from build123d import *

# Parameters (mm, degrees)
SKETCH1_R             = 20
SKETCH1_R_2           = 15
BOSS_EXTRUDE1_DEPTH   = 60
BOSS_EXTRUDE1_2_DEPTH = 60
BOSS_EXTRUDE2_START   = -50
BOSS_EXTRUDE2_DEPTH   = 40


with BuildPart() as part:
    # Sketch1 → Boss-Extrude1 (new body)
    with BuildSketch(Plane.XY):
        Circle(SKETCH1_R)
        Circle(SKETCH1_R_2, mode=Mode.SUBTRACT)
    extrude(amount=BOSS_EXTRUDE1_DEPTH)



with BuildPart() as body_2:
    # Sketch1 → Boss-Extrude1 2 (new body)
    with BuildSketch(Plane.XY):
        with Locations((390, 0)):
            Circle(SKETCH1_R)
        with Locations((390, 0)):
            Circle(SKETCH1_R_2, mode=Mode.SUBTRACT)
    extrude(amount=BOSS_EXTRUDE1_2_DEPTH)


with BuildPart() as part_1:
    add(part.part)

    add(body_2.part)  # Boss-Extrude2 merges body 2
    # Sketch2 → Boss-Extrude2 (add)
    with BuildSketch(Plane.XY.offset(60).offset(BOSS_EXTRUDE2_START)):
        with BuildLine():
            Line((0, -30), (390, -30))
            ThreePointArc((390, -30), (420, 0), (390, 30))
            Line((390, 30), (0, 30))
            ThreePointArc((0, 30), (-30, 0), (0, -30))
        make_face()
        with BuildLine():
            Line((0, 20), (390, 20))
            ThreePointArc((390, 20), (410, 0), (390, -20))
            Line((390, -20), (0, -20))
            ThreePointArc((0, -20), (-20, 0), (0, 20))
        make_face(mode=Mode.SUBTRACT)
    extrude(amount=BOSS_EXTRUDE2_DEPTH)


solid = part_1.part
Build history of the part. All positions in model axes, mm. A direction names the side the tool comes from. Round coordinates to 2 decimals unless told otherwise and drop trailing zeros. Write each loop counter-clockwise with the first axis right and the second up, starting at its lowest first coordinate (ties: lowest second). Pieces come first, ordered by that corner, then holes. Notation, with made-up numbers: M -12,80.5 L 46,80.5 A20 ccw 46,100.5 Z; hole C 7,33.5 d1. An arc over 180 degrees is marked long. Answer as a JSON object with one key per item and string values. Group by question number.
(1) Cut at C-C (y = 0). Give the cut face in (x, z), and give its area (3 significant figures).
(2) Flat gauge pins, fed straight in: pin 1 (6 mm diameter, centred on y = 13.5, z = 25.5, fed in from -X); pin 2 (6 mm diameter, centred on y = 6.5, z = 49, fed in from -X); pin 3 (1.5 mm diameter, centred on x = 270, y = -20.5, fed in from +Z). Where does each tip first touch, or does it go through?
(3) Cut at A-A (x = 97.5). Give the cut face in (y, z).
(4) Mould opens along X. For faces 3 (the cylindrical face through (-14.985, 0.66, 29.58)), 4 (the flat face through (198, 30, 30)), 5 (the cylindrical face through (-29.993, 0.66, 29.72)) say: pulls with the +X half, pulls with the -X half, needs draft (parallel to the pull), parting line crosses it, or undercut.
(5) Drill centre lines: L1, parallel to Y at x = 236.5, z = 32; L2, parallel to X at y = -9.5, z = 51; L3, parallel to Z at x = 5.5, y = -26.5. Where is each one in solid material? Low to high.
(6) Which spindle directions (+Z, -Z, +X, -X, +Y, -Y) get a long thin tool onto all of the face, cutting with end or side? Do faces 1 (the flat face through (192, -30, 30)), 2 (the flat face through (192, 20, 30)). Say none if no direction does.
(7) Cut at B-B (z = 45). Give the cut face in (x, y), and give its area (3 significant figures).
Responses:
{
 "1": {"outline": "M -30,10 L -20,10 L -20,0 L -15,0 L -15,60 L -20,60 L -20,50 L -30,50 Z; M 15,0 L 20,0 L 20,60 L 15,60 Z; M 370,0 L 375,0 L 375,60 L 370,60 Z; M 405,0 L 410,0 L 410,10 L 420,10 L 420,50 L 410,50 L 410,60 L 405,60 Z", "area": "2,000 mm2"},
 "2": {"pin 1": "stops at x = -28.1", "pin 2": "stops at x = -29.8", "pin 3": "stops at z = 50"},
 "3": {"outline": "M -30,10 L -20,10 L -20,50 L -30,50 Z; M 20,10 L 30,10 L 30,50 L 20,50 Z"},
 "4": {"face 3": "undercut", "face 4": "needs draft", "face 5": "pulls with the -X half"},
 "5": {"L1": "y = -30 to -20, 20 to 30", "L2": "x = -17.6 to -11.61, 11.61 to 17.6, 372.4 to 378.39, 401.61 to 407.6", "L3": "z = 10 to 50"},
 "6": {"face 1": "+Z, -Z, +X, -X, -Y", "face 2": "+Z, -Z"},
 "7": {"outline": "M 0,-30 L 390,-30 A30 ccw 390,30 L 0,30 A30 ccw Z; hole C 0,0 d30; hole M 0,-20 L 390,-20 A20 cw 390,20 L 0,20 A20 cw Z; hole C 390,0 d30", "area": "10,500 mm2"}
}
